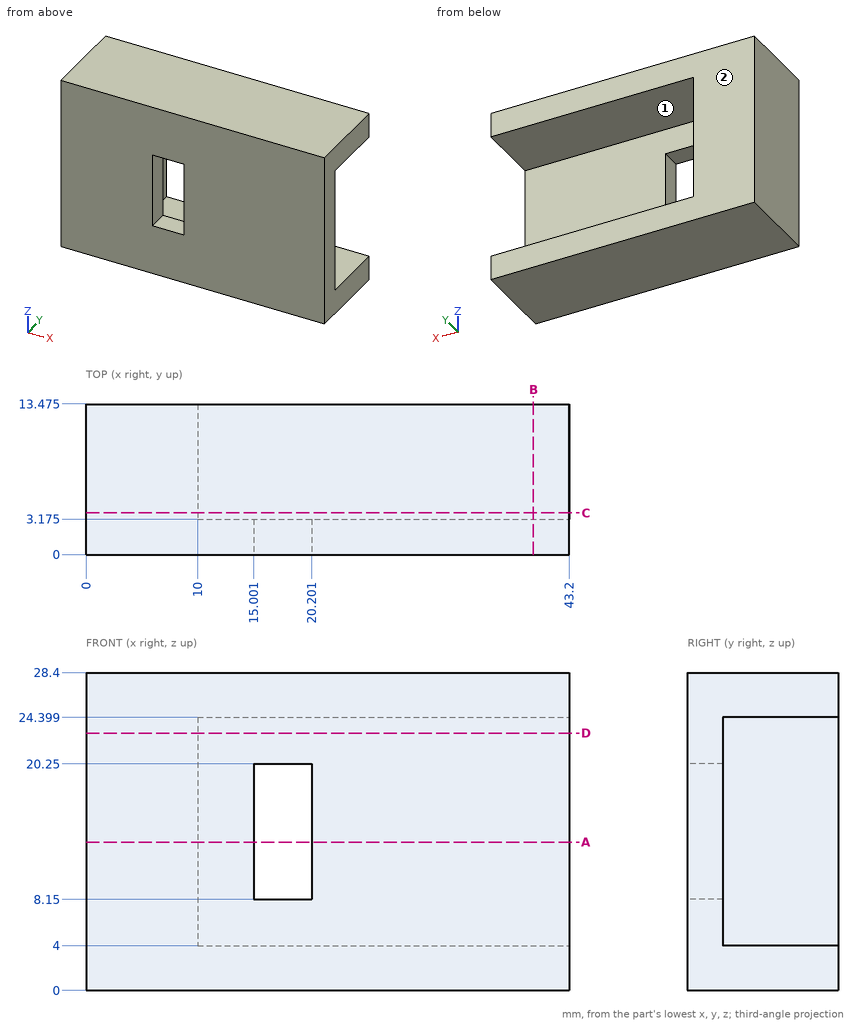
The figure shows three views and two pictorial views of one solid part (mm, origin at its lowest corner). Answer the questions. A direction names the side the tool comes from. Give positions to 0.01 mm unless a question says otherwise; leave off trailing zeros. Order: outer loops, then holes, each group sorted by start corner. A loop starts at its lowest first (then second) coordinate and runs counter-clockwise, first axis right, second up. Notation, with made-up numbers: (-4.75, 47.5) - (24.25, 47.5) arc R29 ccw to (24.25, 68.5) - close; hole circle Ø11 at (78.25, -33.75). An arc over 180 degrees is marked (long way). Answer as CSV lines item,"result".
Q1. A cutting plane is placed at A-A, the plane z = 13.25. Determine the outline of the cut face in (x, y) (1 decimal), and give its area (3 significant figures).
Answer key:
outline,"(0, 0) - (15, 0) - (15, 3.2) - (10, 3.2) - (10, 13.5) - (0, 13.5) - close; (20.2, 0) - (43.2, 0) - (43.2, 3.2) - (20.2, 3.2) - close"
area,"224 mm^2"
Q2. Each of these flat-tipped pins is pushed along its axis until it touches: pin 1 Ø5 at (y, z) = (6, 13) entering from +X; pin 2 Ø5 at (x, z) = (17, 18) entering from +Y (1 decimal). Where does it stop, or does it pass through?
Answer key:
pin 1,"stops at x = 10"
pin 2,"stops at y = 3.2"
Q3. A cutting plane is placed at C-C, the plane y = 3.75. Determine the outline of the cut face in (x, z).
Answer key:
outline,"(0, 0) - (43.2, 0) - (43.2, 4) - (10, 4) - (10, 24.4) - (43.2, 24.4) - (43.2, 28.4) - (0, 28.4) - close"
Q4. A cutting plane is placed at D-D, the plane z = 23. Determine the outline of the cut face in (x, y) (1 decimal), and give its area (3 significant figures).
Answer key:
outline,"(0, 0) - (43.2, 0) - (43.2, 3.2) - (10, 3.2) - (10, 13.5) - (0, 13.5) - close"
area,"240 mm^2"
Q5. A cutting plane is placed at B-B, the plane x = 40. Determine the outline of the cut face in (y, z) (1 decimal).
Answer key:
outline,"(0, 0) - (13.5, 0) - (13.5, 4) - (3.2, 4) - (3.2, 24.4) - (13.5, 24.4) - (13.5, 28.4) - (0, 28.4) - close"
Q6. Which of the six approach directions +Z, -Z, +X, -X, +Y, -Y give full straight-line access (tool end or side, diameter ignored) to the marked faces 1 and 2?
Answer key:
face 1,"+X, +Y"
face 2,"+Z, -Z, +X, -X, +Y"
Q7. Straight lines are drawn through the part: L1, parallel to Z at x = 15.5, y = 8.25; L2, parallel to X at y = 2.5, z = 8.75; L3, parallel to Y at x = 13.5, z = 15 (1 decimal). For each, find the intervals that lie inside material, in ascending order.
Answer key:
L1,"z = 0 to 4, 24.4 to 28.4"
L2,"x = 0 to 15, 20.2 to 43.2"
L3,"y = 0 to 3.2"
